The listing builds one solid part. Answer for the finished solid, in the listing's coordinates (mm). Round coordinates to 2 decimals unless told otherwise and drop trailing zeros. Order: outer loops, then holes, each group sorted by start corner. A loop starts at its lowest first (then second) coordinate and runs counter-clockwise, first axis right, second up. Notation, with made-up numbers: (62, 31) -> (98, 31) arc R23 cw to (98, 52) -> close; hole circle Ø9 at (-20.75, -26). An arc over 180 degrees is marked (long way). Return JSON: item names as keys, results as strings. Group by question number.
(1) The part is cut by section B-B (z = 224.8). Determine the outline of the cut face in (x, y).
(2) The part is cut by section C-C (y = -1). Determine the outline of the cut face in (x, z).
(3) This flat-tipped pin is pushed along its axis until it touches: pin 1 (10 mm diameter, centred on x = 3, z = 223, fed in from +Y). Where does it stop, or does it pass through?
(4) The part is cut by section A-A (x = 0). Determine the outline of the cut face in (y, z), plus the area to 3 significant figures.
(5) Consider line 1 (Z direction, x = 0, y = -11.5); line 2 (X direction, y = -12, z = 224); line 3 (Z direction, x = 0, y = -8.5). Determine where each line is inside the solid, lowest interval first. Write a range as [from, to].
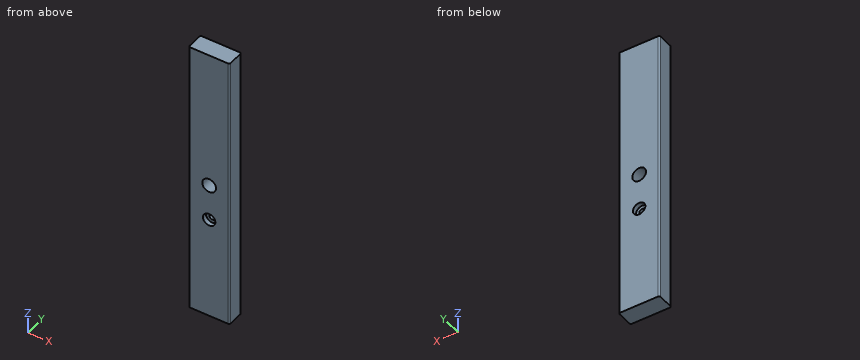
from build123d import *

# Parameters (mm, degrees)
BOSS_EXTRUDE1_DEPTH = 609.6
SKETCH2_R           = 15
SKETCH2_R_2         = 6.35
CUT_EXTRUDE1_DEPTH  = 613.404745654
SKETCH3_R           = 13.5001
CUT_EXTRUDE2_DEPTH  = 10


with BuildPart() as part:
    # Sketch1 → Boss-Extrude1 (new body)
    with BuildSketch(Plane.XY):
        with BuildLine():
            Line((41.45, -19.05), (-41.45, -19.05))
            ThreePointArc((-41.45, -19.05), (-43.571320344, -18.171320344), (-44.45, -16.05))
            Line((-44.45, -16.05), (-44.45, 16.05))
            ThreePointArc((-44.45, 16.05), (-43.571320344, 18.171320344), (-41.45, 19.05))
            Line((-41.45, 19.05), (41.45, 19.05))
            ThreePointArc((41.45, 19.05), (43.571320344, 18.171320344), (44.45, 16.05))
            Line((44.45, 16.05), (44.45, -16.05))
            ThreePointArc((44.45, -16.05), (43.571320344, -18.171320344), (41.45, -19.05))
        make_face()
    extrude(amount=BOSS_EXTRUDE1_DEPTH)

    # Sketch2 → Cut-Extrude1 (cut, through all)
    with BuildSketch(Plane(origin=(0, 19.05, 0), x_dir=(1, 0, 0), z_dir=(0, 1, 0))):
        with Locations(Location((0, -304.8, 0), (0, 0, 180))):
            Circle(SKETCH2_R)
        with Locations(Location((0, -224.8, 0), (0, 0, 180))):
            Circle(SKETCH2_R_2)
    extrude(amount=-CUT_EXTRUDE1_DEPTH, mode=Mode.SUBTRACT)

    # Sketch3 → Cut-Extrude2 (cut)
    with BuildSketch(Plane(origin=(0, 19.05, 0), x_dir=(1, 0, 0), z_dir=(0, 1, 0))):
        with Locations(Location((0, -224.8, 0), (0, 0, 180))):
            Circle(SKETCH3_R)
    cut_extrude2 = extrude(amount=-CUT_EXTRUDE2_DEPTH, mode=Mode.SUBTRACT)

    # Mirror1: Cut-Extrude2 across plane
    add(cut_extrude2.mirror(Plane.ZX), mode=Mode.SUBTRACT)


solid = part.part
Answer below:
{
 "1": {"outline": "(-44.45, -16.05) arc R3 ccw to (-41.45, -19.05) -> (-13.5, -19.05) -> (-13.5, -9.05) -> (-6.35, -9.05) -> (-6.35, 9.05) -> (-13.5, 9.05) -> (-13.5, 19.05) -> (-41.45, 19.05) arc R3 ccw to (-44.45, 16.05) -> close; (6.35, -9.05) -> (13.5, -9.05) -> (13.5, -19.05) -> (41.45, -19.05) arc R3 ccw to (44.45, -16.05) -> (44.45, 16.05) arc R3 ccw to (41.45, 19.05) -> (13.5, 19.05) -> (13.5, 9.05) -> (6.35, 9.05) -> close"},
 "2": {"outline": "(-44.45, 0) -> (44.45, 0) -> (44.45, 609.6) -> (-44.45, 609.6) -> close; hole circle Ø30 at (0, 304.8); hole circle Ø12.7 at (0, 224.8)"},
 "3": {"pin 1": "stops at y = 9.05"},
 "4": {"outline": "(-19.05, 0) -> (19.05, 0) -> (19.05, 211.3) -> (9.05, 211.3) -> (9.05, 218.45) -> (-9.05, 218.45) -> (-9.05, 211.3) -> (-19.05, 211.3) -> close; (-19.05, 238.3) -> (-9.05, 238.3) -> (-9.05, 231.15) -> (9.05, 231.15) -> (9.05, 238.3) -> (19.05, 238.3) -> (19.05, 289.8) -> (-19.05, 289.8) -> close; (-19.05, 319.8) -> (19.05, 319.8) -> (19.05, 609.6) -> (-19.05, 609.6) -> close", "area": "21,300 mm²"},
 "5": {"line 1": "z = [0, 211.3], [238.3, 289.8], [319.8, 609.6]", "line 2": "x = [-44.45, -13.48], [13.48, 44.45]", "line 3": "z = [0, 218.45], [231.15, 289.8], [319.8, 609.6]"}
}
